```python
from build123d import *

# Parameters (mm, degrees)
SKETCH2_W          = 65
SKETCH2_H          = 160
BASE_DEPTH         = 25
SKETCH3_W          = 57
SKETCH3_H          = 152
INSIDE_SPACE_DEPTH = 21
SKETCH4_W          = 57
SKETCH4_H          = 4
BATTERY_WALL_DEPTH = 21
FILLET1_R          = 4


with BuildPart() as part:
    # Sketch2 → Base (new body)
    with BuildSketch(Plane(origin=(0, 0, 0), x_dir=(1, 0, 0), z_dir=(0, 1, 0))):
        Rectangle(SKETCH2_W, SKETCH2_H)
    extrude(amount=BASE_DEPTH)

    # Sketch3 → Inside Space (cut)
    with BuildSketch(Plane(origin=(0, 25, 0), x_dir=(1, 0, 0), z_dir=(0, 1, 0))):
        Rectangle(SKETCH3_W, SKETCH3_H)
    extrude(amount=-INSIDE_SPACE_DEPTH, mode=Mode.SUBTRACT)

    # Sketch4 → Battery Wall (add)
    with BuildSketch(Plane(origin=(0, 4, 0), x_dir=(1, 0, 0), z_dir=(0, 1, 0))):
        with Locations((0, 34)):
            Rectangle(SKETCH4_W, SKETCH4_H)
    extrude(amount=BATTERY_WALL_DEPTH)

    # Fillet1
    fillet1_edges = [part.edges().sort_by_distance(p)[0] for p in [
        (0, 0, -80),
        (32.5, 0, 0),
        (0, 0, 80),
        (-32.5, 0, 0),
        (-32.5, 12.5, -80),
        (32.5, 12.5, -80),
        (32.5, 12.5, 80),
        (-32.5, 12.5, 80),
    ]]
    fillet(fillet1_edges, radius=FILLET1_R)


solid = part.part
```
Geometry check sheet. Reference: the model listing, model coordinates, mm. A direction names the side the tool comes from. Give positions to 0.01 mm unless a question says otherwise; leave off trailing zeros. Loops run counter-clockwise (first coordinate to the right, second up) from the corner with the lowest first, then second, coordinate; pieces in that order, holes last. Notation, with made-up numbers: M 76,50.5 L 123,50.5 A16 cw 123,64.5 Z; hole C 28,-17.5 d7. An arc over 180 degrees is marked long. Write item = value, one per line.
(1) Sectioned sample at C-C, the plane x = 3.5. Record the cut outline in (y, z), plus the area to 3 significant figures.
Answer below:
outline = M 0,-76 A4 ccw 4,-80 L 25,-80 L 25,-76 L 4,-76 L 4,-36 L 25,-36 L 25,-32 L 4,-32 L 4,76 L 25,76 L 25,80 L 4,80 A4 ccw 0,76 Z
area = 885 mm2
(2) Release check for a two-part mould opening along Z. For faces 3 (the face through (0.399, 1.203, -78.859)), 4 (the face through (0, 14, -36)), 5 (the face through (-31.359, 1.203, -1.064)) record: released by +Z, released by -Z, zero draft, split by the parting line, or undercut.
Answer below:
face_3 = released by -Z
face_4 = undercut
face_5 = zero draft
(3) Tool access check on faces 1 (the face through (28.5, 15, 23)), 2 (the face through (0.399, 1.203, 78.859)). Record the directions out of +Z, -Z, +X, -X, +Y, -Y that give a thin tool (end or side, any length) a straight path to the whole face; none if there is none.
Answer below:
face_1 = +Y
face_2 = +Z, +X, -X, -Y
(4) Material ranges on line 1 (Z direction, x = 4, y = 14.5); line 2 (X direction, y = 16.75, z = -13.5); line 3 (Y direction, x = -14.5, z = -28.5), recorded low to high. Write a range as [from, to].
Answer below:
line_1 = [-80, -76], [-36, -32], [76, 80]
line_2 = [-32.5, -28.5], [28.5, 32.5]
line_3 = [0, 4]
(5) Sectioned sample at A-A, the plane y = 17. Record the cut outline in (x, z).
Answer below:
outline = M -32.5,-76 A4 ccw -28.5,-80 L 28.5,-80 A4 ccw 32.5,-76 L 32.5,76 A4 ccw 28.5,80 L -28.5,80 A4 ccw -32.5,76 Z; hole M -28.5,-76 L 28.5,-76 L 28.5,-36 L -28.5,-36 Z; hole M -28.5,-32 L 28.5,-32 L 28.5,76 L -28.5,76 Z
(6) Sectioned sample at B-B, the plane z = 47. Record the cut outline in (x, y).
Answer below:
outline = M -32.5,4 A4 ccw -28.5,0 L 28.5,0 A4 ccw 32.5,4 L 32.5,25 L 28.5,25 L 28.5,4 L -28.5,4 L -28.5,25 L -32.5,25 Z
(7) Gauge pin test, flat end, axial feed: pin 1 Ø12 at (x, z) = (2.5, -52.5) entering from +Y. Record the tip position at first contact, or that the pin passes through.
Answer below:
pin_1 = 4
